CAD build for the part. Positions are in the model's coordinates, mm. A direction names the side the tool comes from. Round coordinates to 2 decimals unless told otherwise and drop trailing zeros. Order: outer loops, then holes, each group sorted by start corner. A loop starts at its lowest first (then second) coordinate and runs counter-clockwise, first axis right, second up. Notation, with made-up numbers: (-39, 57.25) -> (14, 57.25) arc R23 cw to (14, 79.25) -> close; hole circle Ø6 at (63.25, 11.25). An arc over 180 degrees is marked (long way). Return JSON: item names as keys, results as strings. Group by question number.
Q1. Which spindle directions (+Z, -Z, +X, -X, +Y, -Y) get a long thin tool onto all of the face, cutting with end or side? Do faces 1 (the flat face through (10, -5, 2)), 2 (the flat face through (0, 0, 0)). Say none if no direction does.
Q2. Cut at C-C (z = 20). Write the cut outline in (x, y), then the cut area to 3 significant figures.
Q3. Cut at D-D (z = 26). Write the cut outline in (x, y).
Q4. Probe line 1 along Z through (x, y) = (-15, -14); line 2 along X through (y, z) = (7.5, 7.5); line 3 along Y through (x, z) = (0.5, 8). List the from-to ranges inside material, lowest first.
Q5. Flat gauge pins, fed straight in: pin 1 (2 mm diameter, centred on x = 6.5, z = 22, fed in from -Y); pin 2 (2 mm diameter, centred on y = 3, z = 13, fed in from -X); pin 3 (1.5 mm diameter, centred on x = -10.5, y = -17, fed in from -Z); pin 4 (4 mm diameter, centred on x = -12, y = 2.5, fed in from +Z). Where does each tip first touch, or does it go through?
Q6. Cut at A-A (y = 0). Write the cut outline in (x, z), then the cut area to 3 significant figures.
from build123d import *

# Parameters (mm, degrees)
F2_R = 2
F3_R = 1
F4_R = 1


with BuildPart() as f1:
    # F0 (on Front) → F1 (revolve)
    with BuildSketch(Plane.XZ):
        Polygon((-25, 0), (0, 0), (0, 46), (-8, 46), (-9.25, 2), (-25, 2), align=None)
    revolve(axis=Axis((0, 0, 23), (0, 0, -1)))

    # F2
    f2_edges = [f1.edges().sort_by_distance(p)[0] for p in [
        (8, 0, 46),
    ]]
    fillet(f2_edges, radius=F2_R)

    # F3
    f3_edges = [f1.edges().sort_by_distance(p)[0] for p in [
        (25, 0, 2),
    ]]
    fillet(f3_edges, radius=F3_R)

    # F4
    f4_edges = [f1.edges().sort_by_distance(p)[0] for p in [
        (9.25, 0, 2),
    ]]
    fillet(f4_edges, radius=F4_R)


solid = f1.part
Solution:
{
 "1": {"face 1": "+Z", "face 2": "-Z, +X, -X, +Y, -Y"},
 "2": {"outline": "circle Ø17.48 at (0, 0)", "area": "240 mm²"},
 "3": {"outline": "circle Ø17.14 at (0, 0)"},
 "4": {"line 1": "z = 0 to 2", "line 2": "x = -5.14 to 5.14", "line 3": "y = -9.07 to 9.07"},
 "5": {"pin 1": "stops at y = -6.72", "pin 2": "stops at x = -8.71", "pin 3": "stops at z = 0", "pin 4": "stops at z = 2"},
 "6": {"outline": "(-25, 0) -> (25, 0) -> (25, 1) arc R1 ccw to (24, 2) -> (10.22, 2) arc R1 cw to (9.22, 2.97) -> (8.06, 44.06) arc R2 ccw to (6.06, 46) -> (-6.06, 46) arc R2 ccw to (-8.06, 44.06) -> (-9.22, 2.97) arc R1 cw to (-10.22, 2) -> (-24, 2) arc R1 ccw to (-25, 1) -> close", "area": "857 mm²"}
}
